Here's the drawing with two shaded views (mm, measured from the low corner). I have some questions. A direction names the side the tool comes from. Round coordinates to 2 decimals unless told otherwise and drop trailing zeros. Write each loop counter-clockwise with the first axis right and the second up, starting at its lowest first coordinate (ties: lowest second). Pieces come first, ordered by that corner, then holes. Notation, with made-up numbers: M 33,80 L 69,80 A24 cw 69,108 Z; hole C 15,67.25 d7. An arc over 180 degrees is marked long. Answer as a JSON object with one key per item and string values. Group by question number.
1) On a 3-axis mill with a long thin cutter (end or side, diameter ignored), from which of +Z, -Z, +X, -X, +Y, -Y can I reach the whole of each face in a straight line? I mean the marked faces 5 and 6. Say none if no direction works.
2) Suppose I cut it at B-B, the plane x = 19. Write out the boundary of the cut face in (y, z).
3) Suppose I cut it at D-D, the plane x = 5. Write out the boundary of the cut face in (y, z), and give its area (3 significant figures).
4) Suppose I cut it at A-A, the plane z = 17.5. Write out the boundary of the cut face in (x, y).
5) Please list where these lines run through material, in increasing order: L1, parallel to X at y = 19, z = 24; L2, parallel to X at y = 24.25, z = 14.5. Write a range as [from, to].
6) If we mould it in two halves opening along X, with no side actions, what happens to the marked faces 1, 2, 3 and 4? For each: +X half, -X half, draft (parallel to the pull), parting line (faces both ways), or undercut.
7) Suppose I cut it at C-C, the plane y = 15.75. Write out the boundary of the cut face in (x, z).
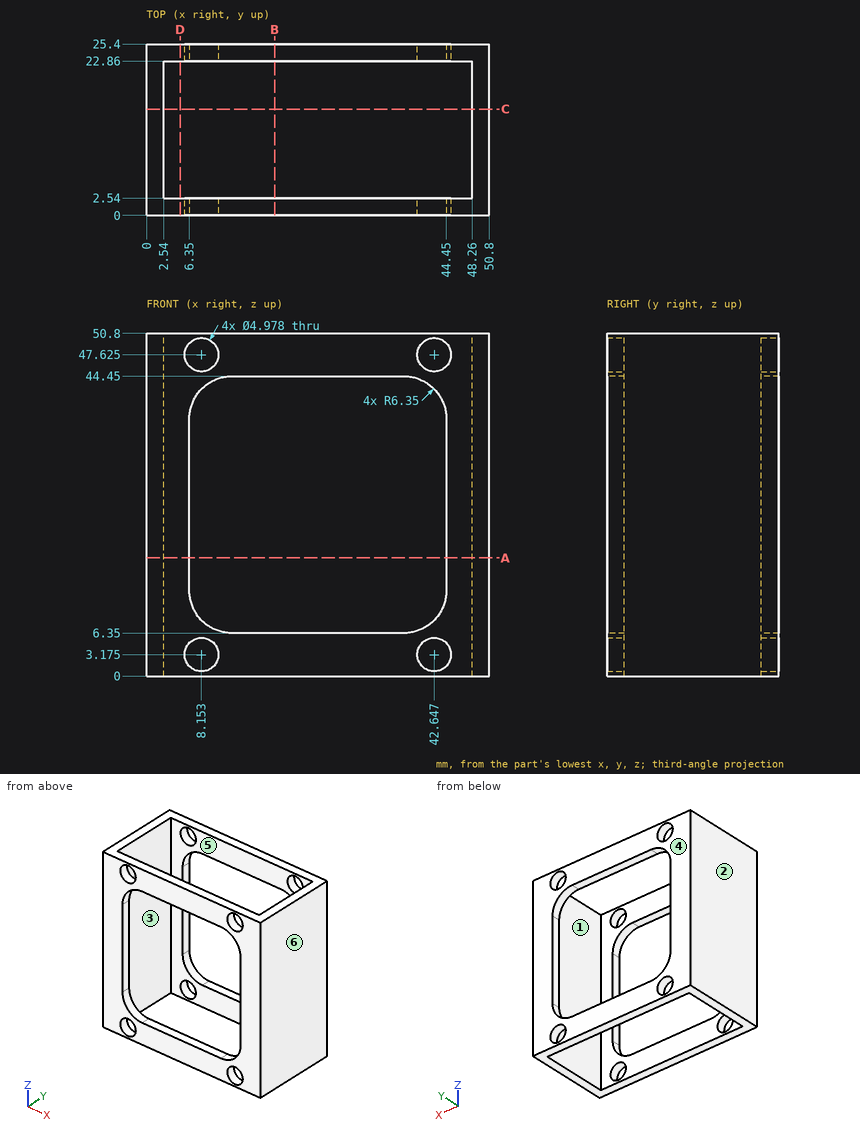
Results:
{
 "1": {"face 5": "+Z, -Z", "face 6": "+Z, -Z, +X, +Y, -Y"},
 "2": {"outline": "M 0,0 L 2.54,0 L 2.54,6.35 L 0,6.35 Z; M 0,44.45 L 2.54,44.45 L 2.54,50.8 L 0,50.8 Z; M 22.86,0 L 25.4,0 L 25.4,6.35 L 22.86,6.35 Z; M 22.86,44.45 L 25.4,44.45 L 25.4,50.8 L 22.86,50.8 Z"},
 "3": {"outline": "M 0,0 L 2.54,0 L 2.54,50.8 L 0,50.8 Z; M 22.86,0 L 25.4,0 L 25.4,50.8 L 22.86,50.8 Z", "area": "258 mm^2"},
 "4": {"outline": "M 0,0 L 6.35,0 L 6.35,2.54 L 2.54,2.54 L 2.54,22.86 L 6.35,22.86 L 6.35,25.4 L 0,25.4 Z; M 44.45,0 L 50.8,0 L 50.8,25.4 L 44.45,25.4 L 44.45,22.86 L 48.26,22.86 L 48.26,2.54 L 44.45,2.54 Z"},
 "5": {"L1": "[0, 2.54], [48.26, 50.8]", "L2": "[0, 6.35], [44.45, 50.8]"},
 "6": {"face 1": "undercut", "face 2": "-X half", "face 3": "undercut", "face 4": "draft"},
 "7": {"outline": "M 0,0 L 2.54,0 L 2.54,50.8 L 0,50.8 Z; M 48.26,0 L 50.8,0 L 50.8,50.8 L 48.26,50.8 Z"}
}
